```python
from build123d import *

# Parameters (mm, degrees)
BOX161_W           = 5
BOX161_H           = 7.45
BOX161_DEPTH       = 1.1
BOX160_W           = 5
BOX160_H           = 7.5
BOX160_DEPTH       = 1.2
CUT078_ROLL_ANGLE  = -90
CUT078_PITCH_ANGLE = -32


with BuildPart() as small_cu_gnd_electrode066:
    # Box161 → Box161 (new body)
    with BuildSketch(Plane.XY.offset(0.05)):
        with Locations((2.5, 3.725)):
            Rectangle(BOX161_W, BOX161_H)
    extrude(amount=BOX161_DEPTH)


with BuildPart() as small_cu_electrode001_long_axis_v007:
    # Box160 → Box160 (new body)
    with BuildSketch(Plane.XY):
        with Locations((2.5, 3.75)):
            Rectangle(BOX160_W, BOX160_H)
    extrude(amount=BOX160_DEPTH)

    # Cut078: cut Small Cu GND Electrode066
    add(small_cu_gnd_electrode066.part, mode=Mode.SUBTRACT)


with BuildPart() as small_cu_electrode001_long_axis_v007_1:
    # Cut078 roll: moved
    add(small_cu_electrode001_long_axis_v007.part.rotate(Axis((0, 0, 0), (1, 0, 0)), CUT078_ROLL_ANGLE))


with BuildPart() as small_cu_electrode001_long_axis_v007_2:
    # Cut078 pitch: moved
    add(small_cu_electrode001_long_axis_v007_1.part.rotate(Axis((0, 0, 0), (0, 1, 0)), CUT078_PITCH_ANGLE))


with BuildPart() as small_cu_electrode001_long_axis_v007_3:
    # Cut078 placement: moved
    add(small_cu_electrode001_long_axis_v007_2.part.moved(Location((6.020438, 2.14, 45.877147))))


solid = small_cu_electrode001_long_axis_v007_3.part
```
CAD build for the part. Positions are in the model's coordinates, mm. Round coordinates to 2 decimals unless told otherwise and drop trailing zeros. Loops run counter-clockwise (first coordinate to the right, second up) from the corner with the lowest first, then second, coordinate; pieces in that order, holes last. Notation, with made-up numbers: (13.25, 16.5) - (21.25, 16.5) arc R36 ccw to (21.25, 51.5) - close; hole circle Ø3 at (66.5, 80.25). An arc over 180 degrees is marked (long way). Return JSON: item names as keys, results as strings. Group by question number.
Q1. Band-saw the part on D-D on z = 41.25. Give the cut face in (x, y).
Q2. Band-saw the part on B-B on x = 9.5. Give the cut face in (y, z).
Q3. Band-saw the part on A-A on z = 44.25. Give the cut face in (x, y), plus the area to 3 significant figures.
Q4. Band-saw the part on C-C on x = 11.25. Give the cut face in (y, z), plus the area to 3 significant figures.
Q5. Flat gauge pin, fed straight in: pin 1 Ø3 at (x, z) = (8.5, 41) entering from +Y. Where does the tip first touch, or does it go through?
Solutions:
{
 "1": {"outline": "(8.91, 2.14) - (12.77, 2.14) - (12.77, 3.34) - (8.91, 3.34) - (8.91, 3.29) - (12.67, 3.29) - (12.67, 2.19) - (8.91, 2.19) - close"},
 "2": {"outline": "(2.14, 40.31) - (2.19, 40.31) - (2.19, 48.05) - (2.14, 48.05) - close; (3.29, 40.31) - (3.34, 40.31) - (3.34, 48.05) - (3.29, 48.05) - close"},
 "3": {"outline": "(7.04, 2.14) - (12.93, 2.14) - (12.93, 2.19) - (7.04, 2.19) - close; (7.04, 3.29) - (12.93, 3.29) - (12.93, 3.34) - (7.04, 3.34) - close", "area": "0.590 mm^2"},
 "4": {"outline": "(2.14, 40.3) - (3.34, 40.3) - (3.34, 46.94) - (3.29, 46.94) - (3.29, 40.36) - (2.19, 40.36) - (2.19, 46.94) - (2.14, 46.94) - close", "area": "0.729 mm^2"},
 "5": {"pin 1": "stops at y = 3.34"}
}
